from build123d import *

# Parameters (mm, degrees)
SKETCH1_W           = 15
SKETCH1_H           = 15
BOSS_EXTRUDE1_DEPTH = 8
SKETCH2_R           = 1
CUT_EXTRUDE1_DEPTH  = 1.5
CUT_EXTRUDE2_DEPTH  = 4
SKETCH4_W           = 4.4
SKETCH4_H           = 4.4
CUT_EXTRUDE3_DEPTH  = 2.75
CUT_EXTRUDE4_DEPTH  = 0.25
FILLET1_R           = 0.75


with BuildPart() as part:
    # Sketch1 → Boss-Extrude1 (new body)
    with BuildSketch(Plane(origin=(0, 0, 0), x_dir=(1, 0, 0), z_dir=(0, 1, 0))):
        Rectangle(SKETCH1_W, SKETCH1_H)
    extrude(amount=BOSS_EXTRUDE1_DEPTH)

    # Sketch2 → Cut-Extrude1 (cut)
    with BuildSketch(Plane.XZ):
        with Locations((-3.889087297, 3.889087297)):
            Circle(SKETCH2_R)
        with Locations((3.889087297, -3.889087297)):
            Circle(SKETCH2_R)
        with Locations((-3.889087297, -3.889087297)):
            Circle(SKETCH2_R)
        with Locations((3.889087297, 3.889087297)):
            Circle(SKETCH2_R)
    extrude(amount=-CUT_EXTRUDE1_DEPTH, mode=Mode.SUBTRACT)

    # Sketch3 → Cut-Extrude2 (cut)
    with BuildSketch(Plane.XZ):
        Polygon((-0.707106781, 0), (-1.75, 1.042893219), (-1.75, -1.042893219), align=None)
        Polygon((-0.707106781, 0), (-1.75, -1.042893219), (-1.75, -1.75), (-1.042893219, -1.75), (0, -0.707106781), align=None)
        Polygon((1.042893219, -1.75), (0, -0.707106781), (-1.042893219, -1.75), align=None)
        Polygon((1.75, -1.042893219), (0.707106781, 0), (0, -0.707106781), (1.042893219, -1.75), (1.75, -1.75), align=None)
        Polygon((1.75, 1.042893219), (0.707106781, 0), (1.75, -1.042893219), align=None)
        Polygon((1.75, 1.75), (1.042893219, 1.75), (0, 0.707106781), (0.707106781, 0), (1.75, 1.042893219), align=None)
        Polygon((1.042893219, 1.75), (-1.042893219, 1.75), (0, 0.707106781), align=None)
        Polygon((0, 0.707106781), (-1.042893219, 1.75), (-1.75, 1.75), (-1.75, 1.042893219), (-0.707106781, 0), align=None)
        Polygon((0.707106781, 0), (0, 0.707106781), (-0.707106781, 0), (0, -0.707106781), align=None)
        Polygon((-2.442893219, 3.15), (-3.15, 3.15), (-3.15, 2.442893219), (-1.75, 1.042893219), (-1.75, 1.75), (-1.042893219, 1.75), align=None)
        Polygon((3.15, 3.15), (2.442893219, 3.15), (1.042893219, 1.75), (1.75, 1.75), (1.75, 1.042893219), (3.15, 2.442893219), align=None)
        Polygon((3.15, -3.15), (3.15, -2.442893219), (1.75, -1.042893219), (1.75, -1.75), (1.042893219, -1.75), (2.442893219, -3.15), align=None)
        Polygon((-1.75, -1.042893219), (-3.15, -2.442893219), (-3.15, -3.15), (-2.442893219, -3.15), (-1.042893219, -1.75), (-1.75, -1.75), align=None)
        with BuildLine():
            Line((-3.15, -2.442893219), (-3.15, 2.442893219))
            Line((-3.15, 2.442893219), (-3.630268251, 2.92316147))
            ThreePointArc((-3.630268251, 2.92316147), (-3.758561104, 2.897642435), (-3.889087297, 2.889087297))
            Line((-3.889087297, 2.889087297), (-3.889087297, -2.889087297))
            ThreePointArc((-3.889087297, -2.889087297), (-3.758561104, -2.897642435), (-3.630268251, -2.92316147))
            Line((-3.630268251, -2.92316147), (-3.15, -2.442893219))
        make_face()
        with BuildLine():
            Line((3.630268251, 2.92316147), (3.15, 2.442893219))
            Line((3.15, 2.442893219), (3.15, -2.442893219))
            Line((3.15, -2.442893219), (3.630268251, -2.92316147))
            ThreePointArc((3.630268251, -2.92316147), (3.758561104, -2.897642435), (3.889087297, -2.889087297))
            Line((3.889087297, -2.889087297), (3.889087297, 2.889087297))
            ThreePointArc((3.889087297, 2.889087297), (3.758561104, 2.897642435), (3.630268251, 2.92316147))
        make_face()
        with BuildLine():
            Line((2.92316147, 3.630268251), (2.442893219, 3.15))
            Line((2.442893219, 3.15), (3.15, 3.15))
            Line((3.15, 3.15), (3.15, 2.442893219))
            Line((3.15, 2.442893219), (3.630268251, 2.92316147))
            ThreePointArc((3.630268251, 2.92316147), (3.181980515, 3.181980515), (2.92316147, 3.630268251))
        make_face()
        with BuildLine():
            Line((-2.92316147, 3.630268251), (-2.442893219, 3.15))
            Line((-2.442893219, 3.15), (2.442893219, 3.15))
            Line((2.442893219, 3.15), (2.92316147, 3.630268251))
            ThreePointArc((2.92316147, 3.630268251), (2.897642435, 3.758561104), (2.889087297, 3.889087297))
            Line((2.889087297, 3.889087297), (-2.889087297, 3.889087297))
            ThreePointArc((-2.889087297, 3.889087297), (-2.897642435, 3.758561104), (-2.92316147, 3.630268251))
        make_face()
        with BuildLine():
            Line((-3.15, -3.15), (-3.15, -2.442893219))
            Line((-3.15, -2.442893219), (-3.630268251, -2.92316147))
            ThreePointArc((-3.630268251, -2.92316147), (-3.181980515, -3.181980515), (-2.92316147, -3.630268251))
            Line((-2.92316147, -3.630268251), (-2.442893219, -3.15))
            Line((-2.442893219, -3.15), (-3.15, -3.15))
        make_face()
        with BuildLine():
            Line((2.442893219, -3.15), (-2.442893219, -3.15))
            Line((-2.442893219, -3.15), (-2.92316147, -3.630268251))
            ThreePointArc((-2.92316147, -3.630268251), (-2.897642435, -3.758561104), (-2.889087297, -3.889087297))
            Line((-2.889087297, -3.889087297), (2.889087297, -3.889087297))
            ThreePointArc((2.889087297, -3.889087297), (2.897642435, -3.758561104), (2.92316147, -3.630268251))
            Line((2.92316147, -3.630268251), (2.442893219, -3.15))
        make_face()
        with BuildLine():
            Line((3.630268251, -2.92316147), (3.15, -2.442893219))
            Line((3.15, -2.442893219), (3.15, -3.15))
            Line((3.15, -3.15), (2.442893219, -3.15))
            Line((2.442893219, -3.15), (2.92316147, -3.630268251))
            ThreePointArc((2.92316147, -3.630268251), (3.181980515, -3.181980515), (3.630268251, -2.92316147))
        make_face()
        with BuildLine():
            Line((-3.15, 2.442893219), (-3.15, 3.15))
            Line((-3.15, 3.15), (-2.442893219, 3.15))
            Line((-2.442893219, 3.15), (-2.92316147, 3.630268251))
            ThreePointArc((-2.92316147, 3.630268251), (-3.181980515, 3.181980515), (-3.630268251, 2.92316147))
            Line((-3.630268251, 2.92316147), (-3.15, 2.442893219))
        make_face()
    extrude(amount=-CUT_EXTRUDE2_DEPTH, mode=Mode.SUBTRACT)

    # Sketch4 → Cut-Extrude3 (cut)
    with BuildSketch(Plane.XZ.offset(-4)):
        Rectangle(SKETCH4_W, SKETCH4_H)
    extrude(amount=CUT_EXTRUDE3_DEPTH, mode=Mode.SUBTRACT)

    # Sketch5 → Cut-Extrude4 (cut)
    with BuildSketch(Plane(origin=(0, 8, 0), x_dir=(1, 0, 0), z_dir=(0, 1, 0))):
        Polygon((4, 0), (-4, 5), (-4, -5), align=None)
    extrude(amount=-CUT_EXTRUDE4_DEPTH, mode=Mode.SUBTRACT)

    # Fillet1
    fillet1_edges = [part.edges().sort_by_distance(p)[0] for p in [
        (0, 0, 1.75),
        (1.75, 0, 0),
        (0, 0, -1.75),
        (-1.75, 0, 0),
    ]]
    fillet(fillet1_edges, radius=FILLET1_R)


solid = part.part
Geometry check sheet. Reference: the model listing, model coordinates, mm. A direction names the side the tool comes from. Give positions to 0.01 mm unless a question says otherwise; leave off trailing zeros. Write each loop counter-clockwise with the first axis right and the second up, starting at its lowest first coordinate (ties: lowest second). Pieces come first, ordered by that corner, then holes. Notation, with made-up numbers: M -7.5,-7 L 38.5,-7 A26 ccw 38.5,32 Z; hole C 33,7 d7. An arc over 180 degrees is marked long. Answer as CSV lines item,"result". Start each with the question number.
Q1. Release check for a two-part mould opening along Z. For faces 1 (the face through (0, 4, -7.5)), 2 (the face through (4.57, 0.74, -4.62)) record: pulls with the +Z half, pulls with the -Z half, needs draft (parallel to the pull), parting line crosses it, or undercut.
Q2. Section check B-B, the plane y = 2.5. Record the cut outline in (x, z).
Q3. Section check C-C, the plane z = 0.25. Record the cut outline in (x, y), then the cut area to 3 significant figures.
Q4. Tool access check on faces 3 (the face through (-1, 7.75, 0)), 4 (the face through (3.15, 2, 0)), 5 (the face through (2.2, 3, 0)). Record the directions out of +Z, -Z, +X, -X, +Y, -Y that give a thin tool (end or side, any length) a straight path to the whole face; none if there is none.
Q5. Section check A-A, the plane x = 2. Record the cut outline in (y, z).
Q6. Section check D-D, the plane x = 0.25. Record the cut outline in (y, z).
Q7. Material ranges on L1, parallel to X at y = 1, z = 0.75; L2, parallel to X at y = 3.75, z = 0.5; L3, parallel to Z at x = -2.25, y = 2.75, recorded low to high.
Geometry says:
1,face 1,"pulls with the -Z half"
1,face 2,"undercut"
2,outline,"M -7.5,-7.5 L 7.5,-7.5 L 7.5,7.5 L -7.5,7.5 Z; M -3.15,-2.44 L -2.2,-1.49 L -2.2,1.49 L -3.15,2.44 Z; M -2.44,-3.15 L 2.44,-3.15 L 1.49,-2.2 L -1.49,-2.2 Z; M -2.44,3.15 L -1.49,2.2 L 1.49,2.2 L 2.44,3.15 Z; M 2.2,-1.49 L 3.15,-2.44 L 3.15,2.44 L 2.2,1.49 Z; hole M -3.89,-2.89 A1 cw -2.89,-3.89 L 2.89,-3.89 A1 cw 3.89,-2.89 L 3.89,2.89 A1 cw 2.89,3.89 L -2.89,3.89 A1 cw -3.89,2.89 Z"
3,outline,"M -7.5,0 L -3.89,0 L -3.89,4 L -3.15,4 L -3.15,0 L -2.5,0 A0.75 ccw -1.75,0.75 L -1.75,1.25 L -2.2,1.25 L -2.2,4 L 2.2,4 L 2.2,1.25 L 1.75,1.25 L 1.75,0.75 A0.75 ccw 2.5,0 L 3.15,0 L 3.15,4 L 3.89,4 L 3.89,0 L 7.5,0 L 7.5,8 L 3.6,8 L 3.6,7.75 L -4,7.75 L -4,8 L -7.5,8 Z"
3,area,"95.5 mm^2"
4,face 3,"+Y"
4,face 4,"-Y"
4,face 5,"none"
5,outline,"M 0,-7.5 L 8,-7.5 L 8,-1.25 L 7.75,-1.25 L 7.75,1.25 L 8,1.25 L 8,7.5 L 0,7.5 L 0,3.89 L 4,3.89 L 4,3.15 L 0,3.15 L 0,2.71 L 4,2.71 L 4,-2.71 L 0,-2.71 L 0,-3.15 L 4,-3.15 L 4,-3.89 L 0,-3.89 Z; M 0.19,-1.29 L 1.25,-1.29 L 1.25,1.29 L 0.19,1.29 Z"
6,outline,"M 0,-7.5 L 8,-7.5 L 8,-2.34 L 7.75,-2.34 L 7.75,2.34 L 8,2.34 L 8,7.5 L 0,7.5 L 0,3.89 L 4,3.89 L 4,3.15 L 0,3.15 L 0,2.5 A0.75 ccw 0.75,1.75 L 1.25,1.75 L 1.25,2.2 L 4,2.2 L 4,-2.2 L 1.25,-2.2 L 1.25,-1.75 L 0.75,-1.75 A0.75 ccw 0,-2.5 L 0,-3.15 L 4,-3.15 L 4,-3.89 L 0,-3.89 Z"
7,L1,"-7.5 to -3.89, -3.15 to -1.75, 1.75 to 3.15, 3.89 to 7.5"
7,L2,"-7.5 to -3.89, -3.15 to -2.2, 2.2 to 3.15, 3.89 to 7.5"
7,L3,"-7.5 to -3.89, -3.15 to -2.96, -1.54 to 1.54, 2.96 to 3.15, 3.89 to 7.5"
